from build123d import *

# Parameters (mm, degrees)
F1_DEPTH = 12
F2_R     = 1.85
F3_DEPTH = 19.151
F4_SIZE  = 1.5


with BuildPart() as f1:
    # F0 (on Front) → F1 (new body)
    with BuildSketch(Plane.XZ):
        with BuildLine():
            Line((-35.8277369916, 41.9945976296), (-39.0277369916, 41.9945976296))
            Line((-39.0277369916, 41.9945976296), (-39.0277369916, 27.5945976296))
            Line((-39.0277369916, 27.5945976296), (-30.5277369916, 27.5945976296))
            ThreePointArc((-30.5277369916, 27.5945976296), (-22.2777369916, 19.3445976296), (-30.5277369916, 11.0945976296))
            Line((-30.5277369916, 11.0945976296), (-39.0277369916, 11.0945976296))
            Line((-39.0277369916, 11.0945976296), (-39.0277369916, -3.3054023704))
            Line((-39.0277369916, -3.3054023704), (-35.8277369916, -3.3054023704))
            Line((-35.8277369916, -3.3054023704), (-35.8277369916, 8.6945976296))
            Line((-35.8277369916, 8.6945976296), (-30.5277369916, 8.6945976296))
            ThreePointArc((-30.5277369916, 8.6945976296), (-19.8777369916, 19.3445976296), (-30.5277369916, 29.9945976296))
            Line((-30.5277369916, 29.9945976296), (-35.8277369916, 29.9945976296))
            Line((-35.8277369916, 29.9945976296), (-35.8277369916, 41.9945976296))
        make_face()
    extrude(amount=F1_DEPTH)

    # F2 (on face) → F3 (cut, through all)
    with BuildSketch(Plane(origin=(-39.0277369916, 0, 0), x_dir=(0, -1, 0), z_dir=(-1, 0, 0))):
        with Locations((6, 35.9945976296)):
            Circle(F2_R)
        with Locations((6, 2.6945976296)):
            Circle(F2_R)
    extrude(amount=-F3_DEPTH, mode=Mode.SUBTRACT)

    # F4
    f4_edges = [f1.edges().sort_by_distance(p)[0] for p in [
        (-35.827737, -4.15, 35.994598),
        (-35.827737, -4.15, 2.694598),
    ]]
    chamfer(f4_edges, length=F4_SIZE)


solid = f1.part
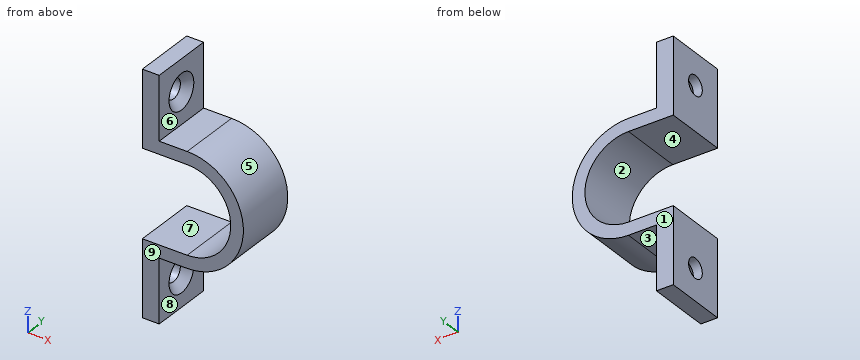
Design review of the part built by this model. Coordinates are the model's own, in mm. Face numbers are marked on the shaded views. A direction names the side the tool comes from. Round coordinates to 2 decimals unless told otherwise and drop trailing zeros. Loops run counter-clockwise (first coordinate to the right, second up) from the corner with the lowest first, then second, coordinate; pieces in that order, holes last. Notation, with made-up numbers: (66, 70.25) - (105, 70.25) arc R15 cw to (105, 94.25) - close; hole circle Ø6 at (10.25, 14). An arc over 180 degrees is marked (long way). One line per question, with ' | ' between items.
1. For L1, parallel to Z at x = -38.25, y = -6; L2, parallel to Z at x = -38, y = -1.25; L3, parallel to Z at x = -33, y = -5.5, list the stretches that pass through material, from the lowest coordinate up. Write a range as [from, to].
Results are:
L1: z = [-3.31, 0.84], [4.54, 11.09], [27.59, 34.14], [37.84, 41.99] | L2: z = [-3.31, 11.09], [27.59, 41.99] | L3: z = [8.69, 11.09], [27.59, 29.99]
2. We need section B-B, the plane y = -6. State the section outline as (x, z) points, and give its area (3 significant figures).
Results are:
outline: (-39.03, -3.31) - (-35.83, -3.31) - (-35.83, -0.66) - (-37.33, 0.84) - (-39.03, 0.84) - close; (-39.03, 4.54) - (-37.33, 4.54) - (-35.83, 6.04) - (-35.83, 8.69) - (-30.53, 8.69) arc R10.65 ccw to (-30.53, 29.99) - (-35.83, 29.99) - (-35.83, 32.64) - (-37.33, 34.14) - (-39.03, 34.14) - (-39.03, 27.59) - (-30.53, 27.59) arc R8.25 cw to (-30.53, 11.09) - (-39.03, 11.09) - close; (-39.03, 37.84) - (-37.33, 37.84) - (-35.83, 39.34) - (-35.83, 41.99) - (-39.03, 41.99) - close | area: 161 mm²
3. We need section A-A, the plane x = -33.75. State the section outline as (y, z) points, and give its area (3 significant figures).
Results are:
outline: (-12, 8.69) - (0, 8.69) - (0, 11.09) - (-12, 11.09) - close; (-12, 27.59) - (0, 27.59) - (0, 29.99) - (-12, 29.99) - close | area: 57.6 mm²
4. We need section D-D, the plane z = 31.5. State the section outline as (x, y) points.
Results are:
outline: (-39.03, -12) - (-35.83, -12) - (-35.83, 0) - (-39.03, 0) - close
5. Clearance check with flat-ended pins moving along their axes: P1, Ø2, axis at y = -3.5, z = 11, coming from the +X side; P2, Ø5, axis at x = -23.5, y = -4.5, coming from the -Z side (3 decimals); P3, Ø5, axis at y = -6, z = 2.69, coming from the +X side; P4, Ø10, axis at x = -32.5, z = 20, coming from the -Y side. State where each tip first meets the part, or that it passes through.
Results are:
P1: stops at x = -22.82 | P2: stops at z = 9.705 | P3: stops at x = -36.67 | P4: passes through
6. For the marked faces 5, 6, 7, 8 and 9, list the 3-axis set-ups (+Z, -Z, +X, -X, +Y, -Y) from which the entire face can be reached by the end or side of a thin tool; tool diameter is ignored.
Results are:
face 5: +X, +Y, -Y | face 6: +Z, +X, +Y, -Y | face 7: -X, +Y, -Y | face 8: -Z, +X, +Y, -Y | face 9: +Z, -Z, +X, -X, -Y
7. Draft analysis for pull direction Z (two halves, no side actions). For the marked faces 1, 2, 3 and 4, state which applies: released by +Z, released by -Z, zero draft, split by the parting line, or undercut.
Results are:
face 1: zero draft | face 2: undercut | face 3: released by -Z | face 4: undercut
8. We need section C-C, the plane y = -11.5. State the section outline as (x, z) points.
Results are:
outline: (-39.03, -3.31) - (-35.83, -3.31) - (-35.83, 8.69) - (-30.53, 8.69) arc R10.65 ccw to (-30.53, 29.99) - (-35.83, 29.99) - (-35.83, 41.99) - (-39.03, 41.99) - (-39.03, 27.59) - (-30.53, 27.59) arc R8.25 cw to (-30.53, 11.09) - (-39.03, 11.09) - close
